from build123d import *

# Parameters (mm, degrees)
SKETCH1_R               = 63.5
BOSS_EXTRUDE1_DEPTH     = 38.1
CUT_EXTRUDE2_DEPTH      = 31.75
SKETCH4_R               = 6.35
BOSS_EXTRUDE2_DEPTH     = 6.35
CUT_EXTRUDE3_DEPTH      = 98.550550998
CUT_EXTRUDE3_DEPTH_BACK = 15.24
SKETCH3_R               = 2.94
CUT_EXTRUDE4_REACH      = 103.798
CUT_EXTRUDE4_END_RADIUS = 2.94
SKETCH5_R               = 1.263861724


with BuildPart() as part:
    # Sketch1 → Boss-Extrude1 (new body)
    with BuildSketch(Plane(origin=(0, 0, 0), x_dir=(1, 0, 0), z_dir=(0, 1, 0))):
        with Locations(Location((0, 0, 0), (0, 0, 90))):
            Circle(SKETCH1_R)
    extrude(amount=BOSS_EXTRUDE1_DEPTH)

    # Sketch2 → Cut-Extrude2 (cut)
    with BuildSketch(Plane(origin=(0, 38.1, 0), x_dir=(1, 0, 0), z_dir=(0, 1, 0))):
        with BuildLine():
            Line((-1.7819572, -9.111319007), (-16.057301334, -50.738697991))
            ThreePointArc((-16.057301334, -50.738697991), (-15.89484722, -52.75977688), (-14.304875125, -54.018005773))
            ThreePointArc((-14.304875125, -54.018005773), (3.484226214, -55.771270092), (20.916794468, -51.817584942))
            ThreePointArc((20.916794468, -51.817584942), (22.337802979, -50.371249564), (22.247447967, -48.345666393))
            Line((22.247447967, -48.345666393), (2.902107489, -8.818689111))
            ThreePointArc((2.902107489, -8.818689111), (0.462316687, -7.400205158), (-1.7819572, -9.111319007))
        make_face()
        with BuildLine():
            Line((8.704163204, -3.229403726), (51.669220951, -12.749274735))
            ThreePointArc((51.669220951, -12.749274735), (53.309221074, -13.941562792), (53.554027291, -15.954327341))
            ThreePointArc((53.554027291, -15.954327341), (45.776114287, -32.048740393), (33.314033776, -44.863677441))
            ThreePointArc((33.314033776, -44.863677441), (31.338979429, -45.322274799), (29.657547842, -44.189164464))
            Line((29.657547842, -44.189164464), (6.012483905, -7.074004722))
            ThreePointArc((6.012483905, -7.074004722), (6.073963109, -4.252498707), (8.704163204, -3.229403726))
        make_face()
        with BuildLine():
            Line((7.951806494, 4.791688532), (42.1830167, 32.447580836))
            ThreePointArc((42.1830167, 32.447580836), (44.13770839, 32.986405118), (45.863985261, 31.922864157))
            ThreePointArc((45.863985261, 31.922864157), (53.597654639, 15.807144497), (55.846795761, -1.926084944))
            ThreePointArc((55.846795761, -1.926084944), (54.973915369, -3.756175388), (53.039658589, -4.3642888))
            Line((53.039658589, -4.3642888), (9.279401997, 0.290179402))
            ThreePointArc((9.279401997, 0.290179402), (7.111791423, 2.097426005), (7.951806494, 4.791688532))
        make_face()
        with BuildLine():
            Line((1.211577307, 9.204541593), (0.932140496, 53.210746228))
            ThreePointArc((0.932140496, 53.210746228), (1.729601044, 55.074937175), (3.637426875, 55.761487836))
            ThreePointArc((3.637426875, 55.761487836), (21.059067856, 51.759927174), (36.325781471, 42.461888801))
            ThreePointArc((36.325781471, 42.461888801), (37.212371773, 40.638400701), (36.481824607, 38.746985345))
            Line((36.481824607, 38.746985345), (5.55874112, 7.435852518))
            ThreePointArc((5.55874112, 7.435852518), (2.794295742, 6.867946156), (1.211577307, 9.204541593))
        make_face()
        with BuildLine():
            Line((-6.440994304, 6.686187096), (-41.020656513, 33.905134408))
            ThreePointArc((-41.020656513, 33.905134408), (-41.980931166, 35.690918215), (-41.328188139, 37.610573848))
            ThreePointArc((-41.328188139, 37.610573848), (-27.33742655, 48.736428979), (-10.549287178, 54.875194214))
            ThreePointArc((-10.549287178, 54.875194214), (-8.570846762, 54.431432191), (-7.547567398, 52.680989231))
            Line((-7.547567398, 52.680989231), (-2.347765198, 8.982177024))
            ThreePointArc((-2.347765198, 8.982177024), (-3.627361626, 6.466762771), (-6.440994304, 6.686187096))
        make_face()
        with BuildLine():
            Line((-9.243365832, -0.867002658), (-52.084062499, -10.931735159))
            ThreePointArc((-52.084062499, -10.931735159), (-54.078965953, -10.569090123), (-55.172834542, -8.861869364))
            ThreePointArc((-55.172834542, -8.861869364), (-55.148281182, 9.013405721), (-49.480527415, 25.966359134))
            ThreePointArc((-49.480527415, 25.966359134), (-47.900042872, 27.236485042), (-45.89348721, 26.94513373))
            Line((-45.89348721, 26.94513373), (-8.486356436, 3.764739028))
            ThreePointArc((-8.486356436, 3.764739028), (-7.317541705, 1.195975121), (-9.243365832, -0.867002658))
        make_face()
        with BuildLine():
            Line((-5.085294358, -7.767321727), (-23.927107102, -47.536785185))
            ThreePointArc((-23.927107102, -47.536785185), (-25.454436367, -48.870358028), (-27.471211214, -48.661144195))
            ThreePointArc((-27.471211214, -48.661144195), (-41.431355264, -37.496895885), (-51.15192129, -22.495673991))
            ThreePointArc((-51.15192129, -22.495673991), (-51.159529717, -20.468090867), (-49.680675096, -19.080957051))
            Line((-49.680675096, -19.080957051), (-8.234548188, -4.287624243))
            ThreePointArc((-8.234548188, -4.287624243), (-5.49746363, -4.975406188), (-5.085294358, -7.767321727))
        make_face()
    extrude(amount=-CUT_EXTRUDE2_DEPTH, mode=Mode.SUBTRACT)

    # Sketch4 → Boss-Extrude2 (add)
    with BuildSketch(Plane.XZ):
        with Locations(Location((0, 0, 0), (0, 0, 90))):
            Circle(SKETCH4_R)
    extrude(amount=BOSS_EXTRUDE2_DEPTH)

    # Sketch3 → Cut-Extrude3 (cut, two sides: drawn at the far end of the back side and taken through both)
    with BuildSketch(Plane.XZ.offset(-CUT_EXTRUDE3_DEPTH_BACK)):
        with Locations(Location((0, 0, 0), (0, 0, 270))):
            Circle(SKETCH3_R)
    extrude(amount=CUT_EXTRUDE3_DEPTH + CUT_EXTRUDE3_DEPTH_BACK, mode=Mode.SUBTRACT)

    # Cut-Extrude4: up to this cylinder (the profile starts outside it)
    cut_extrude4_end = Plane(origin=(0, -3.175, 0), z_dir=(0, 1, 0)) * Cylinder(CUT_EXTRUDE4_END_RADIUS, 214.476, mode=Mode.PRIVATE)
    # Sketch5 → Cut-Extrude4 (cut, up to the surface)
    with BuildSketch(Plane.XY.offset(6.35), mode=Mode.PRIVATE) as cut_extrude4_sk1:
        with Locations((0, -3.175)):
            Circle(SKETCH5_R)
    cut_extrude4_tool1 = extrude(cut_extrude4_sk1.sketch, amount=-CUT_EXTRUDE4_REACH, mode=Mode.PRIVATE) - cut_extrude4_end
    add(cut_extrude4_tool1.solids().sort_by_distance((0, -3.175, 6.35))[0], mode=Mode.SUBTRACT)


solid = part.part
Geometry check sheet. Reference: the model listing, model coordinates, mm. Give positions to 0.01 mm unless a question says otherwise; leave off trailing zeros. Order: outer loops, then holes, each group sorted by start corner. A loop starts at its lowest first (then second) coordinate and runs counter-clockwise, first axis right, second up.
1. Draft check along Z on faces 1 (the face through (1, -6.35, 3)), 2 (the face through (-30.36, 22.45, 5.83)), 3 (the face through (3.86, -3.13, -5.04)). Enter one of: pulls with the +Z half, pulls with the -Z half, needs draft (parallel to the pull), parting line crosses it, or undercut.
Completed:
face 1: needs draft
face 2: undercut
face 3: parting line crosses it
2. Sectioned sample at B-B (y = 30). State how many separate pieces and enclosed holes the cut face has, then the cut area to 3 significant figures.
Completed:
separate pieces: 1
enclosed holes: 7
area: 5,130 mm2
3. Sectioned sample at A-A (z = -44). Record the boundary of the cut face in (x, y), then the cut area to 3 significant figures.
Completed:
outline: (-45.78, 0) - (45.78, 0) - (45.78, 38.1) - (34.45, 38.1) - (34.45, 6.35) - (0.99, 6.35) - (0.99, 38.1) - (-6.51, 38.1) - (-6.51, 6.35) - (-34.45, 6.35) - (-34.45, 38.1) - (-45.78, 38.1) - close
area: 1,540 mm2
4. Scan lines: line 1 (X direction, y = 17, z = -36); line 2 (Z direction, x = 26.5, y = 13); line 3 (Z direction, x = 28.5, y = 10.5) (3 decimals). Record each from-to range of solid material in increasing order.
Completed:
line 1: x = -52.31 to -41.99, -5.56 to 1.04, 33.77 to 52.31
line 2: z = -57.71 to -49.2, -28.64 to -19.78, 1.54 to 7.17, 39.23 to 57.71
line 3: z = -56.745 to -48.066, -30.665 to -21.393, 1.754 to 7.616, 42.372 to 56.745
5. Sectioned sample at C-C (z = 33). Record the boundary of the cut face in (x, y), then the cut area to 3 significant figures.
Completed:
outline: (-54.25, 0) - (54.25, 0) - (54.25, 38.1) - (45.1, 38.1) - (45.1, 6.35) - (22.53, 6.35) - (22.53, 38.1) - (14.74, 38.1) - (14.74, 6.35) - (-9.97, 6.35) - (-9.97, 38.1) - (-17.04, 38.1) - (-17.04, 6.35) - (-45.1, 6.35) - (-45.1, 38.1) - (-54.25, 38.1) - close
area: 1,740 mm2
6. Depth check by flat-ended pin: pin 1 (5 mm diameter, centred on x = 45.5, y = 17, fed in from +Z); pin 2 (13.5 mm diameter, centred on x = -29.5, z = 32, fed in from +Y); pin 3 (1.5 mm diameter, centred on x = -35, y = 10, fed in from -Z). Enter the tip coordinate at first touch or a pass-through.
Completed:
pin 1: stops at z = 46.73
pin 2: stops at y = 6.35
pin 3: stops at z = -53.47
